```python
from build123d import *

# Parameters (mm, degrees)
F0_W     = 20
F0_H     = 20
F1_DEPTH = 15
F1_TAPER = 3
F2_R     = 2
F4_W     = 20
F4_H     = 20
F5_DEPTH = 15
F5_TAPER = 3
F6_R     = 2
F9_DEPTH = 3


with BuildPart() as f1:
    # F0 (on Top) → F1 (new body)
    with BuildSketch(Plane.XY):
        with Locations((1.3560000807, 2.0036636425)):
            Rectangle(F0_W, F0_H)
    extrude(amount=F1_DEPTH, taper=F1_TAPER)

    # F2
    f2_edges = [f1.edges().sort_by_distance(p)[0] for p in [
        (1.356, 11.217547, 15),
        (10.962941, 11.610605, 7.500009),
        (-8.250942, 11.610605, 7.5),
        (10.569883, 2.003664, 15),
        (10.962942, -7.603278, 7.5),
        (-8.250942, -7.603278, 7.5),
        (-7.857883, 2.003664, 15),
        (1.356, -7.21022, 15),
    ]]
    fillet(f2_edges, radius=F2_R)


with BuildPart() as f5:
    # F4 (on Top) → F5 (new body)
    with BuildSketch(Plane.XY):
        with Locations((2.0978832617, 1.2803806274)):
            Rectangle(F4_W, F4_H)
    extrude(amount=F5_DEPTH, taper=F5_TAPER)

    # F6
    f6_edges = [f5.edges().sort_by_distance(p)[0] for p in [
        (-7.509058, 10.887322, 7.5),
        (11.704824, 10.887322, 7.500009),
        (11.704825, -8.326561, 7.5),
        (11.311767, 1.280381, 15),
        (2.097883, 10.494264, 15),
        (-7.116, 1.280381, 15),
        (2.097883, -7.933503, 15),
        (-7.509058, -8.326561, 7.5),
    ]]
    fillet(f6_edges, radius=F6_R)

    # F8 (on face) → F9 (cut)
    with BuildSketch(Plane.XY.offset(15)):
        with BuildLine():
            Line((-0.838498876, -5.4438896477), (1.5617019963, -5.4438896477))
            Line((1.5617019963, -5.4438896477), (3.9619028685, -5.4438896477))
            Line((3.9619028685, -5.4438896477), (3.1234039925, -4.8952721991))
            Line((3.1234039925, -4.8952721991), (2.6932252222, -4.8952721991))
            Line((2.6932252222, -4.8952721991), (2.6932252222, 5.0484170206))
            Line((2.6932252222, 5.0484170206), (2.1446079481, 5.0484170206))
            ThreePointArc((2.1446079481, 5.0484170206), (2.0965612153, 6.3076305978), (1.5617019963, 7.4486183003))
            ThreePointArc((1.5617019963, 7.4486183003), (1.0268427772, 6.3076305978), (0.9787960444, 5.0484170206))
            Line((0.9787960444, 5.0484170206), (0.4301787703, 5.0484170206))
            Line((0.4301787703, 5.0484170206), (0.4301787703, -4.8952721991))
            Line((0.4301787703, -4.8952721991), (0, -4.8952721991))
            Line((0, -4.8952721991), (-0.838498876, -5.4438896477))
        make_face()
    extrude(amount=-F9_DEPTH, mode=Mode.SUBTRACT)


solid = f5.part
```
Source: CAD feature listing. Evaluate the final solid. Frame: model axes, mm. A direction names the side the tool comes from. Coordinates: 2 decimals unless noted, no trailing zeros. Loops run counter-clockwise (first coordinate to the right, second up) from the corner with the lowest first, then second, coordinate; pieces in that order, holes last. Notation, with made-up numbers: (4, -16.75) -> (29, -16.75) arc R18 ccw to (29, 18.25) -> close; hole circle Ø3 at (53, 33.5). An arc over 180 degrees is marked (long way). One line per item, written item: value. Start each with the question number.
Q1. Contact query for flat-ended pins moving along their axis: P1, Ø3.5, axis at y = 2.5, z = 13, coming from the +X side; P2, Ø3, axis at x = 10, z = 3, coming from the +Y side; P3, Ø4, axis at x = -2.5, z = 10, coming from the -Y side. Output: stop coordinate, or through.
Q2. Section query D-D, the plane x = -0.5. Return the cut outline in (y, z), and give its area (3 significant figures).
Q3. Section query B-B, the plane z = 14.25. Return the cut outline in (x, y).
Q4. Mould query, pull axis X, two halves, no side actions, for faces 3 (the face through (3.549, -5.173, 13.521)), 4 (the face through (1.995, 9.988, 14.436)), 5 (the face through (10.806, 1.383, 14.436)). Classes: pulls with the +X half, pulls with the -X half, needs draft (parallel to the pull), parting line crosses it, or undercut.
Q5. Section query A-A, the plane y = -2.5. Return the cut outline in (x, z).
Q6. Set-up query: faces 1 (the face through (2.693, 0, 14)), 2 (the face through (-6.984, -7.77, 6.657)). Return all of +Z, -Z, +X, -X, +Y, -Y with unobstructed straight access to the full face (end or side cutting, diameter ignored); none if empty.
Q7. Line query: line 1 along X through (y, z) = (-1, 13.5); line 2 along Y through (x, z) = (0.5, 14.25); line 3 along Z through (x, y) = (1.5, -3). Output: solid intervals per line, ascending.
Q8. Section query C-C, the plane x = 8.75. Return the cut outline in (y, z).
Results:
1. P1: x = 11.51
1. P2: y = 11.2
1. P3: y = -8.3
2. outline: (-8.72, 0) -> (11.28, 0) -> (10.59, 13.1) arc R2 ccw to (8.6, 15) -> (-5.22, 15) -> (-5.22, 12) -> (-5.44, 12) -> (-5.44, 15) -> (-6.04, 15) arc R2 ccw to (-8.03, 13.1) -> close
2. area: 286 mm^2
3. outline: (-6.78, -6.04) arc R1.56 ccw to (-5.22, -7.6) -> (9.41, -7.6) arc R1.56 ccw to (10.98, -6.04) -> (10.98, 8.6) arc R1.56 ccw to (9.41, 10.16) -> (-5.22, 10.16) arc R1.56 ccw to (-6.78, 8.6) -> close; hole (-0.84, -5.44) -> (3.96, -5.44) -> (3.12, -4.9) -> (2.69, -4.9) -> (2.69, 5.05) -> (2.14, 5.05) arc R3.17 ccw to (1.56, 7.45) arc R3.17 ccw to (0.98, 5.05) -> (0.43, 5.05) -> (0.43, -4.9) -> (0, -4.9) -> close
4. face 3: undercut
4. face 4: needs draft
4. face 5: pulls with the +X half
5. outline: (-7.9, 0) -> (12.1, 0) -> (11.41, 13.1) arc R2 ccw to (9.41, 15) -> (2.69, 15) -> (2.69, 12) -> (0.43, 12) -> (0.43, 15) -> (-5.22, 15) arc R2 ccw to (-7.22, 13.1) -> close
6. face 1: +Z
6. face 2: +Z, -X, -Y
7. line 1: -7.15 to 0.43, 2.69 to 11.35
7. line 2: -7.6 to -5.44, 5.05 to 10.16
7. line 3: 0 to 12
8. outline: (-8.72, 0) -> (11.28, 0) -> (10.59, 13.1) arc R2 ccw to (8.6, 15) -> (-6.04, 15) arc R2 ccw to (-8.03, 13.1) -> close
